Design review of the part built by this model. Coordinates are the model's own, in mm. Face numbers are marked on the shaded views. Coordinates: 2 decimals unless noted, no trailing zeros. Write each loop counter-clockwise with the first axis right and the second up, starting at its lowest first coordinate (ties: lowest second). Pieces come first, ordered by that corner, then holes. Notation, with made-up numbers: (53, 60.25) -> (79, 60.25) arc R14 cw to (79, 82.25) -> close; hole circle Ø9 at (79, 40.5). An arc over 180 degrees is marked (long way). Answer in a Markdown table with one row per item. Add a question column.
Item 1: Take a section at D-D, the plane z = -23.5. Write out the cut boundary in (x, y).
Item 2: Take a section at C-C, the plane y = 100.5. Write out the cut boundary in (x, z).
Item 3: Take a section at A-A, the plane z = -9.5. Write out the cut boundary in (x, y), and give its area (3 significant figures).
Item 4: Take a section at B-B, the plane x = -11. Write out the cut boundary in (y, z), and give its area (3 significant figures).
Item 5: Clearance check with flat-ended pins moving along their axes: P1, Ø1.5, axis at y = 24, z = -4.5, coming from the +X side; P2, Ø8, axis at x = -14.5, y = 150.5, coming from the +Z side; P3, Ø5, axis at y = 23, z = -16, coming from the +X side. State where each tip first meets the part, or that it passes through.
Item 6: Draft analysis for pull direction X (two halves, no side actions). For the marked faces 1 and 2, state which applies: released by +X, released by -X, zero draft, split by the parting line, or undercut.
Item 7: To check wall thickness, follow line 1 (X direction, y = 76.5, z = 0); line 2 (Z direction, x = 28.5, y = 101.5); line 3 (Z direction, x = 16, y = 93). State the ranges of each line that lie inside material, in increasing order.
from build123d import *

# Parameters (mm, degrees)
SCHIZZO1_R                   = 37.5
ESTRUSIONE_ESTRUSIONE1_DEPTH = 200
TAGLIO_ESTRUSIONE2_DEPTH     = 207.911816966
SMUSSO3_SIZE                 = 20
RACCORDO1_R                  = 10


with BuildPart() as part:
    # Schizzo1 → Estrusione-Estrusione1 (new body)
    with BuildSketch(Plane(origin=(0, 0, 0), x_dir=(-1, 0, 0), z_dir=(0, 1, 0))):
        with Locations(Location((0, 0, 0), (0, 0, 90))):
            Circle(SCHIZZO1_R)
    extrude(amount=ESTRUSIONE_ESTRUSIONE1_DEPTH)

    # Schizzo2 → Taglio-Estrusione2 (cut, through all)
    with BuildSketch(Plane(origin=(0, 200, 0), x_dir=(-1, 0, 0), z_dir=(0, 1, 0))):
        with BuildLine():
            ThreePointArc((36.5, 0), (-8.482219535, 35.500731707), (-32.557641192, -16.5))
            Line((-32.557641192, -16.5), (32.557641192, -16.5))
            ThreePointArc((32.557641192, -16.5), (35.500731707, -8.482219535), (36.5, 0))
        make_face()
    extrude(amount=-TAGLIO_ESTRUSIONE2_DEPTH, mode=Mode.SUBTRACT)

    # Smusso3
    smusso3_edges = [part.edges().sort_by_distance(p)[0] for p in [
        (0, 0, -16.5),
        (0, 200, -16.5),
    ]]
    chamfer(smusso3_edges, length=SMUSSO3_SIZE)

    # Raccordo1
    raccordo1_edges = [part.edges().sort_by_distance(p)[0] for p in [
        (0, 20, -16.5),
        (0, 180, -16.5),
    ]]
    fillet(raccordo1_edges, radius=RACCORDO1_R)


solid = part.part
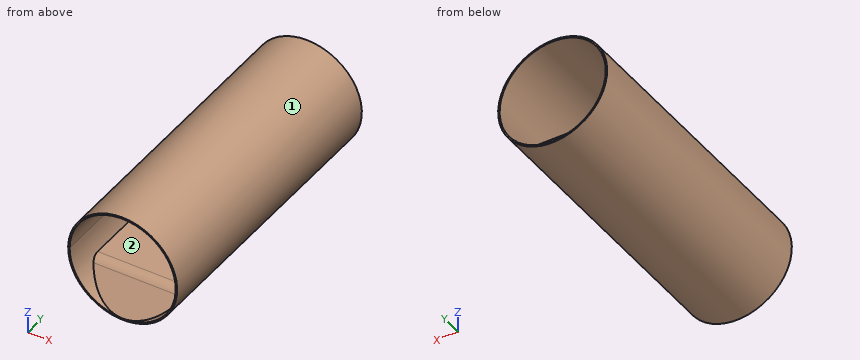
Answers:
| question | item | result |
|---|---|---|
| 1 | outline | (-29.22, 0) -> (-27.93, 0) -> (-27.93, 13) -> (27.93, 13) -> (27.93, 0) -> (29.22, 0) -> (29.22, 200) -> (27.93, 200) -> (27.93, 187) -> (-27.93, 187) -> (-27.93, 200) -> (-29.22, 200) -> close |
| 2 | outline | circle Ø75 at (0, 0); hole (-32.56, -16.5) -> (32.56, -16.5) arc R36.5 ccw (long way) to start |
| 3 | outline | (-36.28, 0) -> (-35.24, 0) -> (-35.24, 200) -> (-36.28, 200) -> close; (35.24, 0) -> (36.28, 0) -> (36.28, 200) -> (35.24, 200) -> close |
| 3 | area | 414 mm^2 |
| 4 | outline | (0, -35.85) -> (200, -35.85) -> (200, -34.8) -> (198.3, -34.8) -> (182.93, -19.43) arc R10 ccw to (175.86, -16.5) -> (24.14, -16.5) arc R10 ccw to (17.07, -19.43) -> (1.7, -34.8) -> (0, -34.8) -> close; (0, 34.8) -> (200, 34.8) -> (200, 35.85) -> (0, 35.85) -> close |
| 4 | area | 3,680 mm^2 |
| 5 | P1 | stops at x = 37.31 |
| 5 | P2 | stops at z = 36 |
| 5 | P3 | stops at x = 34.99 |
| 6 | face 1 | split by the parting line |
| 6 | face 2 | undercut |
| 7 | line 1 | x = -37.5 to -36.5, 36.5 to 37.5 |
| 7 | line 2 | z = -24.37 to -16.5, 22.8 to 24.37 |
| 7 | line 3 | z = -33.92 to -16.5, 32.81 to 33.92 |
